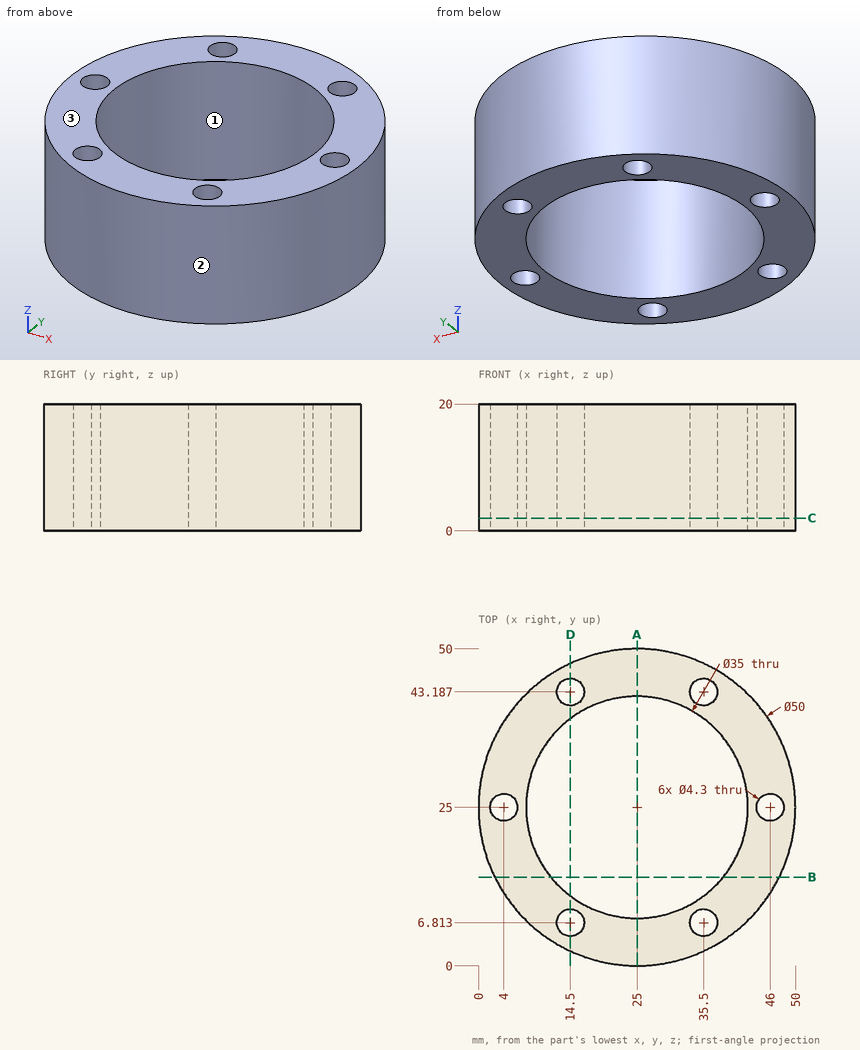
Source: three-view drawing plus pictorial views. Frame: mm from the lowest corner of the part. Round coordinates to 2 decimals unless told otherwise and drop trailing zeros. Write each loop counter-clockwise with the first axis right and the second up, starting at its lowest first coordinate (ties: lowest second). Pieces come first, ordered by that corner, then holes. Notation, with made-up numbers: M 82,-0.75 L 102,-0.75 A37 cw 102,36.25 Z; hole C -8.75,-36.75 d6. An arc over 180 degrees is marked long. One line per item, written item: value. Start each with the question number.
Item 1: Section query B-B (y = 14). Return the cut outline in (x, z).
Item 2: Ray query, L1, parallel to X at y = 5.5, z = 13 (1 decimal); L2, parallel to Y at x = 14.5, z = 5 (1 decimal); L3, parallel to X at y = 5, z = 5.5 (1 decimal). Return the intervals inside material, ascending. Write a range as from..to.
Item 3: Mould query, pull axis X, two halves, no side actions, for the marked faces 1, 2 and 3. Classes: pulls with the +X half, pulls with the -X half, needs draft (parallel to the pull), parting line crosses it, or undercut.
Item 4: Section query C-C (z = 2). Return the cut outline in (x, y).
Item 5: Section query A-A (x = 25). Return the cut outline in (y, z), plus the area to 3 significant figures.
Item 6: Section query D-D (x = 14.5). Return the cut outline in (y, z).
Item 7: Pin query (flat end, axial travel): pin 1 (2.5 mm diameter, centred on x = 46, y = 25, fed in from +Z); pin 2 (2 mm diameter, centred on x = 26.5, z = 3.5, fed in from -Y) (1 decimal); pin 3 (6 mm diameter, centred on y = 15.5, z = 12, fed in from -X); pin 4 (4 mm diameter, centred on y = 39.5, z = 16.5, fed in from +X). Return the tip coordinate at first contact, or that it passes through.
Result set:
1. outline: M 2.55,0 L 11.39,0 L 11.39,20 L 2.55,20 Z; M 38.61,0 L 47.45,0 L 47.45,20 L 38.61,20 Z
2. L1: x = 9.4..12.8, 16.2..33.8, 37.2..40.6
2. L2: y = 2.3..4.7, 9..11, 39..41, 45.3..47.7
2. L3: x = 10..13.3, 15.7..34.3, 36.7..40
3. face 1: undercut
3. face 2: parting line crosses it
3. face 3: needs draft
4. outline: C 25,25 d50; hole C 4,25 d4.3; hole C 25,25 d35; hole C 14.5,6.81 d4.3; hole C 14.5,43.19 d4.3; hole C 35.5,6.81 d4.3; hole C 35.5,43.19 d4.3; hole C 46,25 d4.3
5. outline: M 0,0 L 7.5,0 L 7.5,20 L 0,20 Z; M 42.5,0 L 50,0 L 50,20 L 42.5,20 Z
5. area: 300 mm²
6. outline: M 2.31,0 L 4.66,0 L 4.66,20 L 2.31,20 Z; M 8.96,0 L 11,0 L 11,20 L 8.96,20 Z; M 39,0 L 41.04,0 L 41.04,20 L 39,20 Z; M 45.34,0 L 47.69,0 L 47.69,20 L 45.34,20 Z
7. pin 1: passes through
7. pin 2: stops at y = 0
7. pin 3: stops at x = 0.86
7. pin 4: stops at x = 46.65
